```python
from build123d import *

# Parameters (mm, degrees)
IZIM1_R                     = 40.8
Y_KSEKLIK_EKSTR_ZYON1_DEPTH = 2.9
KES_EKSTR_ZYON1_DEPTH       = 16
KES_EKSTR_ZYON1_DEPTH_BACK  = 7.9
IZIM2_R                     = 9.8
KES_EKSTR_ZYON2_DEPTH       = 1.26
KES_EKSTR_ZYON3_DEPTH       = 21
KES_EKSTR_ZYON3_DEPTH_BACK  = 18.26
IZIM4_R                     = 40.8
IZIM4_R_2                   = 20.4


with BuildPart() as part:
    # Çizim1 → Yükseklik-Ekstrüzyon1 (new body)
    with BuildSketch(Plane(origin=(0, 0, 0), x_dir=(1, 0, 0), z_dir=(0, 1, 0))):
        with Locations(Location((0, 0, 0), (0, 0, 270))):
            Circle(IZIM1_R)
    extrude(amount=Y_KSEKLIK_EKSTR_ZYON1_DEPTH)

    # Çizim2 → Kes-Ekstrüzyon1 (cut, two sides: drawn at the far end of the back side and taken through both)
    with BuildSketch(Plane(origin=(0, 2.9, 0), x_dir=(1, 0, 0), z_dir=(0, 1, 0)).offset(-KES_EKSTR_ZYON1_DEPTH_BACK)):
        with Locations(Location((0, 0, 0), (0, 0, 270))):
            Circle(IZIM2_R)
    extrude(amount=KES_EKSTR_ZYON1_DEPTH + KES_EKSTR_ZYON1_DEPTH_BACK, mode=Mode.SUBTRACT)

    # Çizim3 → Kes-Ekstrüzyon2 (cut)
    with BuildSketch(Plane(origin=(0, 2.9, 0), x_dir=(1, 0, 0), z_dir=(0, 1, 0))):
        Polygon((6, 0), (6, 43.137439927), (-6, 43.137439927), (-6, 0), (-6, -43.926883272), (6, -43.926883272), align=None)
    extrude(amount=-KES_EKSTR_ZYON2_DEPTH, mode=Mode.SUBTRACT)

    # Çizim4 → Kes-Ekstrüzyon3 (cut, two sides: drawn at the far end of the back side and taken through both)
    with BuildSketch(Plane(origin=(0, 2.9, 0), x_dir=(1, 0, 0), z_dir=(0, 1, 0)).offset(-KES_EKSTR_ZYON3_DEPTH_BACK)):
        Circle(IZIM4_R)
        with Locations(Location((0, 0, 0), (0, 0, 72.895364823))):
            Circle(IZIM4_R_2, mode=Mode.SUBTRACT)
    extrude(amount=KES_EKSTR_ZYON3_DEPTH + KES_EKSTR_ZYON3_DEPTH_BACK, mode=Mode.SUBTRACT)


solid = part.part
```
Geometry check sheet. Reference: the model listing, model coordinates, mm. A direction names the side the tool comes from. Round coordinates to 2 decimals unless told otherwise and drop trailing zeros. Order: outer loops, then holes, each group sorted by start corner. A loop starts at its lowest first (then second) coordinate and runs counter-clockwise, first axis right, second up. Notation, with made-up numbers: (17.25, 82.5) - (51.25, 82.5) arc R25 ccw to (51.25, 101.5) - close; hole circle Ø6 at (-16, 65). An arc over 180 degrees is marked (long way). Use a Markdown table: item, result. Add a question column.
(1) Sectioned sample at D-D, the plane z = -13. Enter the section's corners in (x, y), and give its area (3 significant figures).
(2) Sectioned sample at A-A, the plane x = 0. Enter the section's corners in (y, z).
(3) Release check for a two-part mould opening along X. For faces 1 (the cylindrical face through (7.103, 1.43, 19.124)), 2 (the flat face through (6, 2, -14)), 3 (the flat face through (-13, 2.9, 0)) record: pulls with the +X half, pulls with the -X half, needs draft (parallel to the pull), parting line crosses it, or undercut.
(4) Depth check by flat-ended pin: pin 1 (0.6 mm diameter, centred on y = 2, z = -15.5, fed in from +X); pin 2 (9.5 mm diameter, centred on x = 0.5, z = 15.5, fed in from +Y); pin 3 (1.4 mm diameter, centred on y = 2, z = 11, fed in from +X). Enter the tip coordinate at first touch or a pass-through.
(5) Sectioned sample at B-B, the plane z = 0. Enter the section's corners in (x, y), and give its area (3 significant figures).
(6) Tool access check on faces 4 (the flat face through (6, 2, 14)), 5 (the cylindrical face through (9.717, 1.107, -1.276)). Record the directions out of +Z, -Z, +X, -X, +Y, -Y that give a thin tool (end or side, any length) a straight path to the whole face; none if there is none.
(7) Sectioned sample at C-C, the plane y = 0.8. Enter the section's corners in (x, z).
(8) Material ranges on line 1 along X through (y, z) = (1.8, 0); line 2 along Y through (x, z) = (-5, 9.5), recorded low to high. Write a range as [from, to].
Answers below:
| question | item | result |
|---|---|---|
| 1 | outline | (-15.72, 0) - (15.72, 0) - (15.72, 2.9) - (6, 2.9) - (6, 1.64) - (-6, 1.64) - (-6, 2.9) - (-15.72, 2.9) - close |
| 1 | area | 76.1 mm² |
| 2 | outline | (0, -20.4) - (1.64, -20.4) - (1.64, -9.8) - (0, -9.8) - close; (0, 9.8) - (1.64, 9.8) - (1.64, 20.4) - (0, 20.4) - close |
| 3 | face 1 | parting line crosses it |
| 3 | face 2 | undercut |
| 3 | face 3 | needs draft |
| 4 | pin 1 | x = 13.61 |
| 4 | pin 2 | y = 1.64 |
| 4 | pin 3 | x = 17.61 |
| 5 | outline | (-20.4, 0) - (-9.8, 0) - (-9.8, 2.9) - (-20.4, 2.9) - close; (9.8, 0) - (20.4, 0) - (20.4, 2.9) - (9.8, 2.9) - close |
| 5 | area | 61.5 mm² |
| 6 | face 4 | +Z, -Z, +Y |
| 6 | face 5 | +Y, -Y |
| 7 | outline | circle Ø40.8 at (0, 0); hole circle Ø19.6 at (0, 0) |
| 8 | line 1 | [-20.4, -9.8], [9.8, 20.4] |
| 8 | line 2 | [0, 1.64] |
